Autodesk Inventor part; units mm, degrees
ref_plane "YZ Plane" through (0, 0, 0) normal (1, 0, 0) x (0, 1, 0)
ref_plane "XZ Plane" through (0, 0, 0) normal (0, 1, 0) x (-1, 0, 0)
ref_plane "XY Plane" through (0, 0, 0) normal (0, 0, 1) x (1, 0, 0)
sketch "Sketch1" plane through (0, 0, 0) normal (0, 1, 0) x (-1, 0, 0)
  line L0 (-1.5875, 0) -> (-1.5875, -25.4)
  line L1 (-1.5875, -25.4) -> (0, -25.4)
  line L2 (0, -25.4) -> (0, 0)
  line L3 (0, 0) -> (50.8, 29.3294)
  line L4 (50.8, 29.3294) -> (50.8, 0)
  line L5 (52.3875, 29.3294) -> (52.3875, -25.4076)
  line L6 (52.3875, -25.4076) -> (50.8, -25.4076)
  line L7 (50.8, -25.4076) -> (50.8, 29.3294)
  line L8 (-0.7937, 1.3748) -> (50.0062, 30.7042)
  arc A0 (52.3875, 29.3294) -> (50.0062, 30.7042) centre (50.8, 29.3294) ccw
  arc A1 (-0.7937, 1.3748) -> (-1.5875, 0) centre (0, 0) ccw
  dimension "d0" = 1.5875
  dimension "d1" = 25.4
  dimension "d5" = 1.5875
  dimension "d6" = 54.737
  dimension "d7" = 1.5875
  dimension "d8" = 1.5875
extrude "Extrusion1" add sketch "Sketch1" along normal blind 25.4
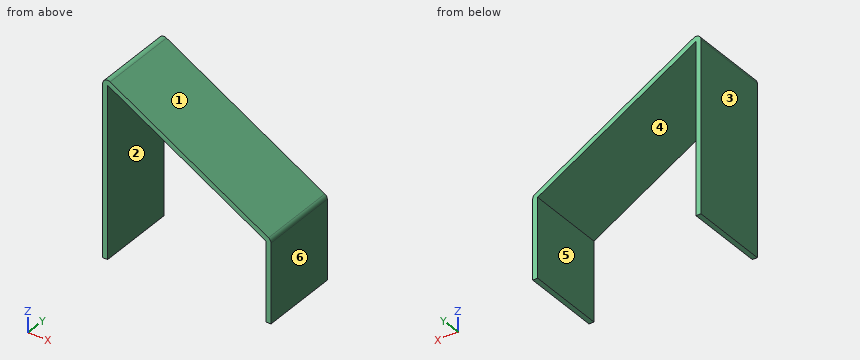
Input: part model. Units: mm. Frame: model coordinates. Face numbers are marked on the shaded views. A direction names the side the tool comes from. Coordinates: 2 decimals unless noted, no trailing zeros. Write each loop counter-clockwise with the first axis right and the second up, starting at its lowest first coordinate (ties: lowest second). Pieces come first, ordered by that corner, then holes.
1) Section C-C on z = 21. Output: boundary loops of the cut face in (x, y).
2) Section A-A on z = -1. Output: boundary loops of the cut face in (x, y).
3) Section B-B on y = 4.5. Output: boundary loops of the cut face in (x, z).
4) Set-up query: the marked faces 1 and 2. Return all of +Z, -Z, +X, -X, +Y, -Y with unobstructed straight access to the full face (end or side cutting, diameter ignored); none if empty.
5) Pin query (flat end, axial travel): pin 1 Ø5 at (x, y) = (-4.5, 22.5) entering from +Z; pin 2 Ø0.5 at (x, y) = (0.5, 13.5) entering from -Z; pin 3 Ø8 at (x, y) = (-46.5, 22) entering from -Z. Return the tip coordinate at first contact, or that it passes through.
6) Material intervals for line 1 along X through (y, z) = (23, -10); line 2 along X through (y, z) = (21.25, 16.5); line 3 along Z through (x, y) = (-39.5, 17), sorted ascending.
7) Section D-D on x = -19.5. Output: boundary loops of the cut face in (y, z), and give its area (3 significant figures).
8) Mould query, pull axis X, two halves, no side actions, for the marked faces 3, 4, 5 and 6. Classes: pulls with the +X half, pulls with the -X half, needs draft (parallel to the pull), parting line crosses it, or undercut.
Check result:
1. outline: (-52.39, 0) - (-50.8, 0) - (-50.8, 25.4) - (-52.39, 25.4) - close; (-36.37, 0) - (-33.2, 0) - (-33.2, 25.4) - (-36.37, 25.4) - close
2. outline: (-52.39, 0) - (-50.8, 0) - (-50.8, 25.4) - (-52.39, 25.4) - close; (0, 0) - (1.59, 0) - (1.59, 25.4) - (0, 25.4) - close
3. outline: (-52.39, -25.41) - (-50.8, -25.41) - (-50.8, 29.33) - (0, 0) - (0, -25.4) - (1.59, -25.4) - (1.59, 0) arc R1.59 ccw to (0.79, 1.37) - (-50.01, 30.7) arc R1.59 ccw to (-52.39, 29.33) - close
4. face 1: +Z, +X, +Y, -Y
4. face 2: -Z, +Y, -Y
5. pin 1: stops at z = 5.87
5. pin 2: stops at z = -25.4
5. pin 3: stops at z = 24.54
6. line 1: x = -52.39 to -50.8, 0 to 1.59
6. line 2: x = -52.39 to -50.8, -28.58 to -25.4
6. line 3: z = 22.81 to 24.64
7. outline: (0, 11.26) - (25.4, 11.26) - (25.4, 13.09) - (0, 13.09) - close
7. area: 46.6 mm2
8. face 3: pulls with the -X half
8. face 4: undercut
8. face 5: undercut
8. face 6: pulls with the +X half
